Could you check a few things on this model? Use its own coordinates, in mm. Face numbers are marked on the shaded views. A direction names the side the tool comes from. Give positions to 0.01 mm unless a question says otherwise; leave off trailing zeros. Order: outer loops, then holes, each group sorted by start corner. A loop starts at its lowest first (then second) coordinate and runs counter-clockwise, first axis right, second up. Notation, with made-up numbers: (50.25, -24) -> (61.25, -24) arc R15 ccw to (61.25, -2) -> close; hole circle Ø4 at (62, -32.75). An arc over 180 degrees is marked (long way). Answer as CSV lines item,"result". Start each with the question number.
(1) I want a section at A-A (y = 18). Please give me the cut outline in (x, z) (3 decimals).
(2) We'd pull the mould along Y, two halves only. Please class the marked faces 3, 4 and 5: released by +Y, released by -Y, zero draft, split by the parting line, or undercut.
(3) I want a section at D-D (y = 7). Please give me the cut outline in (x, z), plus the area to 3 significant figures.
(4) Will these pins go through, and if not, where does the flat tip stop? pin 1 Ø1.5 at (y, z) = (57, 4.5) entering from -X; pin 2 Ø1.5 at (y, z) = (15, -7.5) entering from +X; pin 3 Ø6 at (x, y) = (59, 44) entering from -Z (3 decimals).
(5) I want a section at C-C (x = 2.5). Please give me the cut outline in (y, z), plus the area to 3 significant figures.
(6) On a 3-axis mill with a long thin cutter (end or side, diameter ignored), from which of +Z, -Z, +X, -X, +Y, -Y can I reach the whole of each face in a straight line? I mean the marked faces 1 and 2. Say none if no direction works.
(7) I need wall thicknesses on L1, parallel to Y at x = 25.5, z = -9.75; L2, parallel to Z at x = 0, y = 83.8; L3, parallel to Y at x = -1, z = 10.75. Which ranges of each line are inside material? Lowest first, please.
(8) I want a section at B-B (z = 0). Please give me the cut outline in (x, y), plus the area to 3 significant figures.
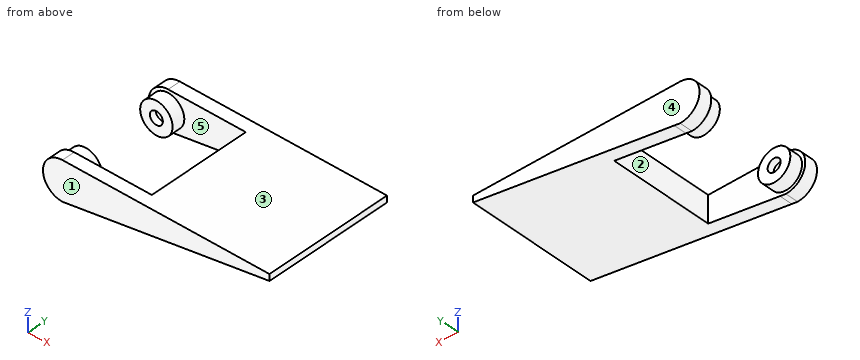
```python
from build123d import *

# Parameters (mm, degrees)
BOSS_EXTRUDE1_DEPTH = 50
SKETCH2_R           = 12.5
CUT_EXTRUDE1_DEPTH  = 40
SKETCH3_R           = 12.5
CUT_EXTRUDE2_DEPTH  = 30
SKETCH4_R           = 5
CUT_EXTRUDE3_DEPTH  = 5


with BuildPart() as part:
    # Sketch1 → Boss-Extrude1 (new body)
    with BuildSketch(Plane(origin=(0, 0, 0), x_dir=(1, 0, 0), z_dir=(0, 1, 0))):
        with BuildLine():
            Line((0, -15), (0, 15))
            ThreePointArc((0, 15), (-15, 0), (0, -15))
        make_face()
        with BuildLine():
            Line((4.575786463, 14.285033365), (0, 15))
            Line((0, 15), (0, -15))
            ThreePointArc((0, -15), (10.606601718, -10.606601718), (15, 0))
            ThreePointArc((15, 0), (12.116864218, 8.842036051), (4.575786463, 14.285033365))
        make_face()
        with BuildLine():
            Line((160, -10), (4.575786463, 14.285033365))
            ThreePointArc((4.575786463, 14.285033365), (12.116864218, 8.842036051), (15, 0))
            ThreePointArc((15, 0), (10.606601718, -10.606601718), (0, -15))
            Line((0, -15), (160, -15))
            Line((160, -15), (160, -10))
        make_face()
    boss_extrude1 = extrude(amount=BOSS_EXTRUDE1_DEPTH)

    # Sketch2 → Cut-Extrude1 (cut)
    with BuildSketch(Plane(origin=(0, 50, 0), x_dir=(1, 0, 0), z_dir=(0, 1, 0))):
        with BuildLine():
            ThreePointArc((15, 0), (10.606601718, -10.606601718), (0, -15))
            Line((0, -15), (60, -15))
            Line((60, -15), (60, 5.625))
            Line((60, 5.625), (4.575786463, 14.285033365))
            ThreePointArc((4.575786463, 14.285033365), (12.116864218, 8.842036051), (15, 0))
        make_face()
        with BuildLine():
            ThreePointArc((0, 15), (-15, 0), (0, -15))
            ThreePointArc((0, -15), (10.606601718, -10.606601718), (15, 0))
            ThreePointArc((15, 0), (12.116864218, 8.842036051), (4.575786463, 14.285033365))
            Line((4.575786463, 14.285033365), (0, 15))
        make_face()
        Circle(SKETCH2_R, mode=Mode.SUBTRACT)
    cut_extrude1 = extrude(amount=-CUT_EXTRUDE1_DEPTH, mode=Mode.SUBTRACT)

    # Sketch3 → Cut-Extrude2 (cut)
    with BuildSketch(Plane(origin=(0, 50, 0), x_dir=(1, 0, 0), z_dir=(0, 1, 0))):
        Circle(SKETCH3_R)
    cut_extrude2 = extrude(amount=-CUT_EXTRUDE2_DEPTH, mode=Mode.SUBTRACT)

    # Sketch4 → Cut-Extrude3 (cut)
    with BuildSketch(Plane(origin=(0, 20, 0), x_dir=(1, 0, 0), z_dir=(0, 1, 0))):
        Circle(SKETCH4_R)
    cut_extrude3 = extrude(amount=-CUT_EXTRUDE3_DEPTH, mode=Mode.SUBTRACT)

    # Mirror1: Boss-Extrude1, Cut-Extrude1, Cut-Extrude2, Cut-Extrude3 across plane
    add(boss_extrude1.mirror(Plane.ZX.offset(50)))
    add(cut_extrude1.mirror(Plane.ZX.offset(50)), mode=Mode.SUBTRACT)
    add(cut_extrude2.mirror(Plane.ZX.offset(50)), mode=Mode.SUBTRACT)
    add(cut_extrude3.mirror(Plane.ZX.offset(50)), mode=Mode.SUBTRACT)


solid = part.part
```
Final values:
1,outline,"circle Ø25 at (0, 0); (60, -5.625) -> (160, 10) -> (160, 15) -> (60, 15) -> close; hole circle Ø10 at (0, 0)"
2,face 3,"zero draft"
2,face 4,"released by +Y"
2,face 5,"undercut"
3,outline,"(0, -15) -> (160, 10) -> (160, 15) -> (0, 15) arc R15 ccw to start"
3,area,"3,150 mm²"
4,pin 1,"x = 60"
4,pin 2,"x = 10.52"
4,pin 3,"z = -5.625"
5,outline,"(0, -14.61) -> (10, -14.61) -> (10, -12.25) -> (20, -12.25) -> (20, -4.33) -> (15, -4.33) -> (15, 4.33) -> (20, 4.33) -> (20, 12.25) -> (10, 12.25) -> (10, 15) -> (0, 15) -> close; (80, -12.25) -> (90, -12.25) -> (90, -14.61) -> (100, -14.61) -> (100, 15) -> (90, 15) -> (90, 12.25) -> (80, 12.25) -> (80, 4.33) -> (85, 4.33) -> (85, -4.33) -> (80, -4.33) -> close"
5,area,"995 mm²"
6,face 1,"+Z, -Z, +X, -X, -Y"
6,face 2,"+Z, -Z"
7,L1,"0 to 10, 90 to 100"
7,L2,"-12.5 to -5, 5 to 12.5"
7,L3,"0 to 20, 80 to 100"
8,outline,"(-15, 0) -> (96, 0) -> (96, 100) -> (-15, 100) -> (-15, 90) -> (-12.5, 90) -> (-12.5, 80) -> (-5, 80) -> (-5, 85) -> (5, 85) -> (5, 80) -> (12.5, 80) -> (12.5, 90) -> (60, 90) -> (60, 10) -> (12.5, 10) -> (12.5, 20) -> (5, 20) -> (5, 15) -> (-5, 15) -> (-5, 20) -> (-12.5, 20) -> (-12.5, 10) -> (-15, 10) -> close"
8,area,"5,500 mm²"
